For this review, use the dimensioned drawing (mm, ordinates from the lowest corner) and the shaded views. A direction names the side the tool comes from. Give positions to 0.01 mm unless a question says otherwise; leave off trailing zeros. Write each loop counter-clockwise with the first axis right and the second up, starting at its lowest first coordinate (ties: lowest second). Pieces come first, ordered by that corner, then holes. Notation, with made-up numbers: M -16.75,-23 L -6.75,-23 A8 ccw -6.75,-14 Z; hole C -19,-20.5 d2. An arc over 180 degrees is marked long. Answer in a Markdown table with one row per item.
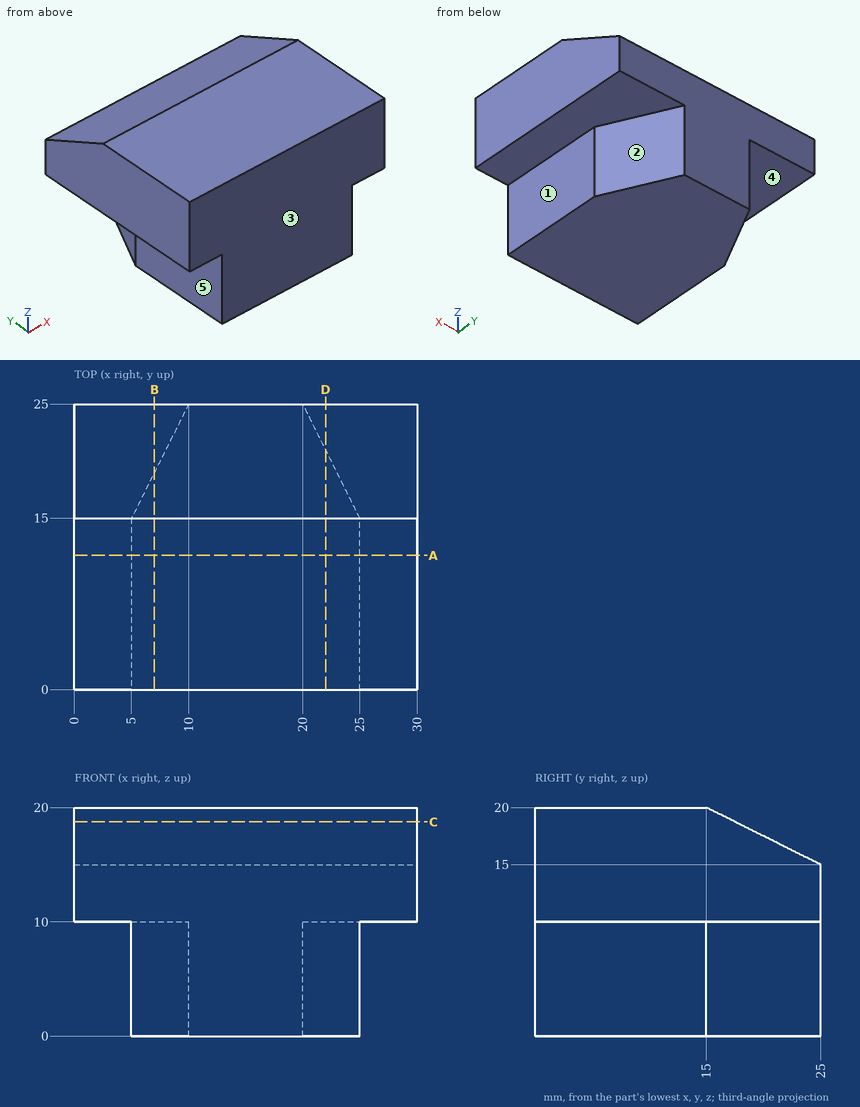
1) Add section A-A (y = 11.75). Write out the cut boundary in (x, z).
Geometry says:
| item | result |
|---|---|
| outline | M 0,10 L 5,10 L 5,0 L 25,0 L 25,10 L 30,10 L 30,20 L 0,20 Z |
2) Add section B-B (x = 7). Write out the cut boundary in (y, z), and give its area (3 significant figures).
Geometry says:
| item | result |
|---|---|
| outline | M 0,0 L 19,0 L 19,10 L 25,10 L 25,15 L 15,20 L 0,20 Z |
| area | 415 mm^2 |
3) Insertion check: P1, Ø3, axis at y = 6.5, z = 4.5, coming from the -X side; P2, Ø4, axis at x = 24, z = 5, coming from the +Y side; P3, Ø5, axis at y = 6.5, z = 4, coming from the +X side. Each pin has a flat end and moves straight along its axis. Give the tip position at first contact, or say it passes through.
Geometry says:
| item | result |
|---|---|
| P1 | x = 5 |
| P2 | y = 21 |
| P3 | x = 25 |
4) To check wall thickness, follow probe 1 along Z at (x, y) = (26, 8.5); probe 2 along X at (y, z) = (12, 8.25); probe 3 along Y at (x, z) = (29, 17.5). State the ranges of each line that lie inside material, in increasing order. Write a range as [from, to].
Geometry says:
| item | result |
|---|---|
| probe 1 | [10, 20] |
| probe 2 | [5, 25] |
| probe 3 | [0, 20] |
5) Add section D-D (x = 22). Write out the cut boundary in (y, z), and give its area (3 significant figures).
Geometry says:
| item | result |
|---|---|
| outline | M 0,0 L 21,0 L 21,10 L 25,10 L 25,15 L 15,20 L 0,20 Z |
| area | 435 mm^2 |
6) For the marked faces 1, 2, 3, 4 and 5, list the 3-axis set-ups (+Z, -Z, +X, -X, +Y, -Y) from which the entire face can be reached by the end or side of a thin tool; tool diameter is ignored.
Geometry says:
| item | result |
|---|---|
| face 1 | -Z, +X, +Y, -Y |
| face 2 | -Z, +X, +Y |
| face 3 | +Z, -Z, +X, -X, -Y |
| face 4 | -Z, -X, +Y |
| face 5 | -Z, -X, +Y, -Y |
7) Add section C-C (z = 18.75). Write out the cut boundary in (x, y).
Geometry says:
| item | result |
|---|---|
| outline | M 0,0 L 30,0 L 30,17.5 L 0,17.5 Z |
